Can you work these out from the model? Positions are in its coordinate system, mm. Give positions to 0.01 mm unless a question says otherwise; leave off trailing zeros. Order: outer loops, then holes, each group sorted by start corner. A loop starts at its lowest first (then second) coordinate and runs counter-clockwise, first axis right, second up. Notation, with made-up numbers: M 23,-0.5 L 44,-0.5 A34 cw 44,35.5 Z; hole C -40,-9.75 d11. An arc over 180 degrees is marked long. Answer as a JSON object with one key per item and string values.
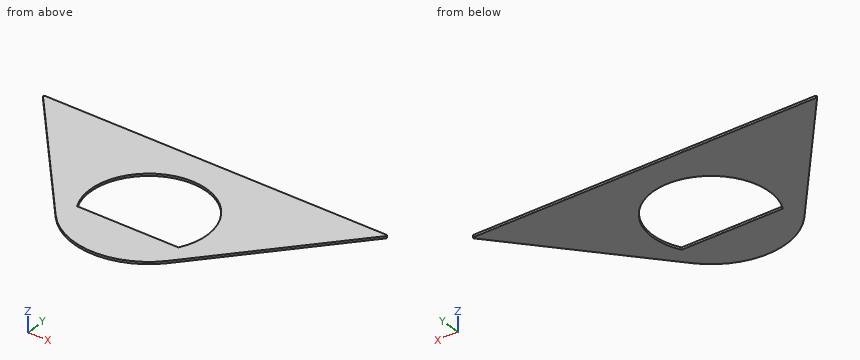
Autodesk Inventor part; units mm, degrees
ref_plane "YZ Plane" through (0, 0, 0) normal (1, 0, 0) x (0, 1, 0)
ref_plane "XZ Plane" through (0, 0, 0) normal (0, 1, 0) x (-1, 0, 0)
ref_plane "XY Plane" through (0, 0, 0) normal (0, 0, 1) x (1, 0, 0)
sketch "Sketch2" plane through (0, 0, 0) normal (0, 0, 1) x (1, 0, 0)
  circle A0 centre (0, 0) radius 67.5
  line L0 (-157.5, 80) -> (-51.2445, -43.9346)
  line L1 (157.5, 80) -> (51.2445, -43.9346)
  line L2 (-157.5, 80) -> (157.5, 80)
  circle A1 centre (0, 0) radius 52.5
  line L3 (46.1655, -25) -> (-46.1655, -25)
  point P0 (0, 80)
  dimension "d11" = 135
  dimension "d12" = 15
  dimension "d13" = 315
  dimension "d14" = 80
  dimension "d15" = 25
extrude "Plate2" add sketch "Sketch2" along normal blind 2 contours A0 | A0 L0 L2 L1 | L3 A1 picked at (-3.1172, -43.6181)
fillet "Corner Round1" radius 1 2 edges at (157.5, 80, 1) (-157.5, 80, 1)
equation "\"d10\" = Thickness"
equation "\"BendRadius\" = Thickness"
equation "\"BendReliefWidth\" = Thickness"
equation "\"BendReliefDepth\" = 0.5 * Thickness"
equation "\"CornerReliefSize\" = 4 * Thickness"
equation "\"MinimumRemnant\" = 2 * Thickness"
equation "\"TransitionRadius\" = BendRadius"
equation "\"JacobiRadiusSize\" = BendRadius"
equation "\"GapSize\" = Thickness"
properties part number "ДМФ 054 фланец лотка v2.0"
1) I want a section at A-A on x = 0. Write out the boundary of the cut face in (y, z).
Results found:
{"outline": "M -67.5,0 L -25,0 L -25,2 L -67.5,2 Z; M 52.5,0 L 80,0 L 80,2 L 52.5,2 Z"}
2) I want a section at D-D on x = 134. Write out the boundary of the cut face in (y, z).
Results found:
{"outline": "M 52.59,0 L 80,0 L 80,2 L 52.59,2 Z"}
3) I need wall thicknesses on L1, parallel to X at y = 25, z = 0.8; L2, parallel to Y at x = 44.5, z = 1.25; L3, parallel to X at y = 0, z = 1.45. Which ranges of each line are inside material? Lowest first, please.
Results found:
{"L1": "x = -110.35 to -46.17, 46.17 to 110.35", "L2": "y = -50.75 to -25, 27.86 to 80", "L3": "x = -88.91 to -52.5, 52.5 to 88.91"}
4) I want a section at B-B on z = 0.3. Write out the boundary of the cut face in (x, y), and give its area (3 significant figures).
Results found:
{"outline": "M -156.08,78.35 L -51.24,-43.93 A67.5 ccw 51.24,-43.93 L 156.08,78.35 A1 ccw 155.33,80 L -155.33,80 A1 ccw Z; hole M -46.17,-25 L 46.17,-25 A52.5 ccw long Z", "area": "20,700 mm²"}
5) I want a section at C-C on y = -22. Write out the boundary of the cut face in (x, z), and give its area (3 significant figures).
Results found:
{"outline": "M -70.05,0 L -47.67,0 L -47.67,2 L -70.05,2 Z; M 47.67,0 L 70.05,0 L 70.05,2 L 47.67,2 Z", "area": "89.5 mm²"}
